Solid Edge part; units mm, degrees
sketch "Sketch1" plane through (0, 0, 0) normal (0, -1, 0) x (1, 0, 0)
  line L0 (2, 0) -> (4, 2)
  line L1 (4, 2) -> (4, 2.3)
  line L2 (4, 2.3) -> (0, 2.3)
  line L3 (0, 2.3) -> (0, -17.7)
  line L4 (0, -17.7) -> (1.5705, -17.7)
  line L5 (1.5705, -17.7) -> (2, -17.2705)
  line L6 (2, -17.2705) -> (2, -2.1)
  line L7 (2, -2.1) -> (1.5705, -2.1)
  line L8 (1.5705, -2.1) -> (1.5705, -2.09)
  line L9 (1.5705, -2.09) -> (2, -2.09)
  line L10 (2, -2.09) -> (2, 0)
  dimension "D1" = 2
  dimension "D2" = 1.5705
revolve "RevolvedProtrusion1" add sketch "Sketch1" angle 360 about axis through (0, 0, 54) along (0, 0, -1)
sketch "Sketch2" plane through (0, 0, 0) normal (0, -1, 0) x (1, 0, 0)
  arc A0 (-1.25, 0.5) -> (0, 0) centre (0, 1.8125) ccw
  line L0 (0, 0.5) -> (0, 0)
  line L1 (-1.25, 0.5) -> (0, 0.5)
revolve "RevolvedCutout1" cut sketch "Sketch2" angle 360 about axis through (0, 0, 54) along (0, 0, -1)
sketch "Sketch3" plane through (0, 0, 2.3) normal (0, 0, 1) x (0, -1, 0)
  line L0 (-1.4434, 0) -> (-0.7217, 1.25)
  line L1 (-0.7217, 1.25) -> (0.7217, 1.25)
  line L2 (0.7217, 1.25) -> (1.4434, 0)
  line L3 (1.4434, 0) -> (0.7217, -1.25)
  line L4 (0.7217, -1.25) -> (-0.7217, -1.25)
  line L5 (-0.7217, -1.25) -> (-1.4434, 0)
extrude "Cutout1" cut sketch "Sketch3" against normal blind 1.8
cosmetic_thread "Thread1"
sketch "Sketch4" plane through (0, 0, 0) normal (1, 0, 0) x (0, 1, 0)
  line L0 (-1.435, 2.3) -> (0, 1.4715)
revolve "RevolvedCutout2" cut sketch "Sketch4" angle 360 about axis through (0, 0, -57) along (0, 0, 1) material side at (0, -0.6925, 1.9291)
fillet "Round1" radius 0.2 1 edges at (-2, 0, 0)
properties material "Stahl"
Input: part model. Units: mm. Frame: model coordinates. A direction names the side the tool comes from. Round coordinates to 2 decimals unless told otherwise and drop trailing zeros. Loops run counter-clockwise (first coordinate to the right, second up) from the corner with the lowest first, then second, coordinate; pieces in that order, holes last. Notation, with made-up numbers: (81.5, 20.5) - (134.5, 20.5) arc R12 ccw to (134.5, 42.5) - close; hole circle Ø6 at (13.25, 82.5). An arc over 180 degrees is marked (long way). One line per item, written item: value. Start each with the question number.
(1) Contact query for flat-ended pins moving along their axis: P1, Ø4, axis at x = -2.5, z = -5, coming from the +Y side; P2, Ø3, axis at x = -1, z = -7, coming from the +Y side; P3, Ø0.7, axis at y = 0, z = 1.5, coming from the +X side. Output: stop coordinate, or through.
(2) Section A-A, the plane z = -11.25. Return loops of the section in (x, y), plus the area to 3 significant figures.
(3) Access query for faces 5 (the cylindrical face through (0, -2, -10)), 6 (the flat face through (1.25, 0, 1)), 7 (the flat face through (2, 0, 2.3)). Directions: +Z, -Z, +X, -X, +Y, -Y. A direction counts if a zero-diameter tool reaches every point of the face in a straight line with its end or side. Return the directions, or none.
(4) Ray query, line 1 (X direction, y = 0, z = -5); line 2 (Z direction, x = -1.5, y = -2); line 3 (X direction, y = 1.5, z = -10.25). Return the intervals inside material, ascending. Write a range as [from, to].
(5) Draft query along Y for faces 1 (the flat face through (0.63, -1.08, 1.41)), 2 (the flat face through (0, 0, -17.7)), 3 (the conical face through (-2.2, 0.1, 0.2)), 4 (the flat face through (-0.63, 1.08, 1.41)). Return one class per face: +Y half, -Y half, draft (parallel to the pull), parting line (faces both ways), or undercut.
Results below:
1. P1: y = 1.94
1. P2: y = 2
1. P3: x = 3.85
2. outline: circle Ø4 at (0, 0)
2. area: 12.6 mm^2
3. face 5: -Z
3. face 6: +Z
3. face 7: +Z, +X, -X, +Y, -Y
4. line 1: [-2, 2]
4. line 2: [0.5, 2.3]
4. line 3: [-1.32, 1.32]
5. face 1: undercut
5. face 2: draft
5. face 3: parting line
5. face 4: undercut
